```python
from build123d import *

# Parameters (mm, degrees)
SKETCH1_R           = 10
SKETCH1_R_2         = 4
BOSS_EXTRUDE1_DEPTH = 1.5
SKETCH2_R           = 6
SKETCH2_R_2         = 4
BOSS_EXTRUDE2_DEPTH = 4
SKETCH3_W           = 30.73076969
SKETCH3_H           = 21.435526278
SKETCH3_R           = 4
BOSS_EXTRUDE3_DEPTH = 3


with BuildPart() as part:
    # Sketch1 → Boss-Extrude1 (new body, symmetric)
    with BuildSketch(Plane(origin=(0, 0, 0), x_dir=(1, 0, 0), z_dir=(0, 1, 0))):
        Circle(SKETCH1_R)
        Circle(SKETCH1_R_2, mode=Mode.SUBTRACT)
    extrude(amount=BOSS_EXTRUDE1_DEPTH, both=True)

    # Sketch2 → Boss-Extrude2 (add)
    with BuildSketch(Plane(origin=(0, 1.5, 0), x_dir=(1, 0, 0), z_dir=(0, 1, 0))):
        Circle(SKETCH2_R)
        Circle(SKETCH2_R_2, mode=Mode.SUBTRACT)
    extrude(amount=BOSS_EXTRUDE2_DEPTH)

    # Sketch3 → Boss-Extrude3 (add)
    with BuildSketch(Plane(origin=(0, 5.5, 0), x_dir=(1, 0, 0), z_dir=(0, 1, 0))):
        Rectangle(SKETCH3_W, SKETCH3_H)
        Circle(SKETCH3_R, mode=Mode.SUBTRACT)
    extrude(amount=BOSS_EXTRUDE3_DEPTH)


solid = part.part
```
Can you work these out from the model? Positions are in its coordinate system, mm. Give positions to 0.01 mm unless a question says otherwise; leave off trailing zeros. Write each loop counter-clockwise with the first axis right and the second up, starting at its lowest first coordinate (ties: lowest second). Pieces come first, ordered by that corner, then holes. Notation, with made-up numbers: (-26.75, -35) -> (32.25, -35) arc R20 cw to (32.25, -10) -> close; hole circle Ø8 at (-38.5, 0). An arc over 180 degrees is marked (long way). One line per item, written item: value.
Q1. Imagine slicing it at B-B on z = 0. Please give me the cut outline in (x, y), and give its area (3 significant figures).
Results found:
outline: (-15.37, 5.5) -> (-6, 5.5) -> (-6, 1.5) -> (-10, 1.5) -> (-10, -1.5) -> (-4, -1.5) -> (-4, 8.5) -> (-15.37, 8.5) -> close; (4, -1.5) -> (10, -1.5) -> (10, 1.5) -> (6, 1.5) -> (6, 5.5) -> (15.37, 5.5) -> (15.37, 8.5) -> (4, 8.5) -> close
area: 120 mm^2
Q2. Imagine slicing it at A-A on x = 0. Please give me the cut outline in (y, z).
Results found:
outline: (-1.5, -10) -> (1.5, -10) -> (1.5, -6) -> (5.5, -6) -> (5.5, -10.72) -> (8.5, -10.72) -> (8.5, -4) -> (-1.5, -4) -> close; (-1.5, 4) -> (8.5, 4) -> (8.5, 10.72) -> (5.5, 10.72) -> (5.5, 6) -> (1.5, 6) -> (1.5, 10) -> (-1.5, 10) -> close
Q3. We'd pull the mould along Y, two halves only. Please class faces 1 (the face through (0, 1.5, 7)), 2 (the face through (-2.17, 0.02, 9.76)), 3 (the face through (-0.1, -1.5, 4.3)), 4 (the face through (-6, 3, 0)): +Y half, -Y half, draft (parallel to the pull), parting line (faces both ways), or undercut.
Results found:
face 1: undercut
face 2: draft
face 3: -Y half
face 4: undercut
Q4. Please list where these lines run through material, in increasing order: line 1 (Y direction, x = 7.5, z = -0.5); line 2 (X direction, y = 4.25, z = 0); line 3 (X direction, y = 1.25, z = 0). Write a range as [from, to].
Results found:
line 1: y = [-1.5, 1.5], [5.5, 8.5]
line 2: x = [-6, -4], [4, 6]
line 3: x = [-10, -4], [4, 10]
Q5. Imagine slicing it at C-C on y = 2.25. Please give me the cut outline in (x, z), and give its area (3 significant figures).
Results found:
outline: circle Ø12 at (0, 0); hole circle Ø8 at (0, 0)
area: 62.8 mm^2
Q6. Imagine slicing it at D-D on z = -4.75. Please give me the cut outline in (x, y).
Results found:
outline: (-15.37, 5.5) -> (-3.67, 5.5) -> (-3.67, 1.5) -> (-8.8, 1.5) -> (-8.8, -1.5) -> (8.8, -1.5) -> (8.8, 1.5) -> (3.67, 1.5) -> (3.67, 5.5) -> (15.37, 5.5) -> (15.37, 8.5) -> (-15.37, 8.5) -> close
Q7. For P1, Ø4, axis at x = 2.5, y = -0.5, coming from the +Z side, with a flat end and sliding along its axis, tell me the tip position at first contact or that it passes through.
Results found:
P1: stops at z = 9.99
